Can you work these out from the model? Positions are in its coordinate system, mm. Give positions to 0.01 mm unless a question says otherwise; leave off trailing zeros. Write each loop counter-clockwise with the first axis right and the second up, starting at its lowest first coordinate (ties: lowest second). Pieces come first, ordered by that corner, then holes.
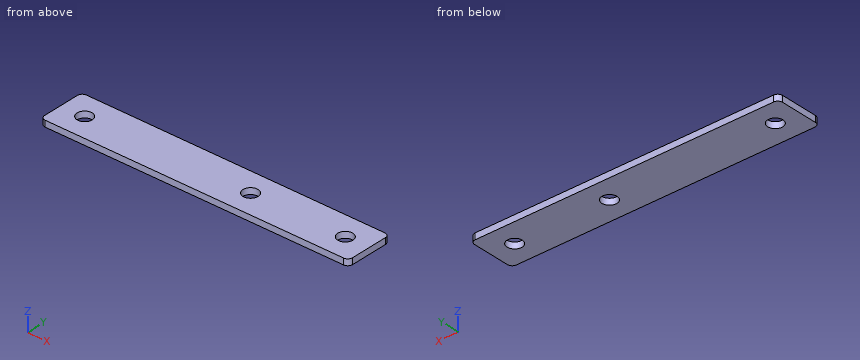
from build123d import *

# Parameters (mm, degrees)
SKETCH_1_W      = 65
SKETCH_1_H      = 10
SKETCH_1_R      = 1.6
EXTRUDE_1_DEPTH = 1.3
FILLET_1_R      = 1


with BuildPart() as part:
    # 草图1 → 凸台-拉伸1 (new body)
    with BuildSketch(Plane.XY):
        with Locations((32.5, 5)):
            Rectangle(SKETCH_1_W, SKETCH_1_H)
        with Locations((60, 5)):
            Circle(SKETCH_1_R, mode=Mode.SUBTRACT)
        with Locations((40, 5)):
            Circle(SKETCH_1_R, mode=Mode.SUBTRACT)
        with Locations((5, 5)):
            Circle(SKETCH_1_R, mode=Mode.SUBTRACT)
    extrude(amount=EXTRUDE_1_DEPTH)

    # 圆角1
    fillet_1_edges = [part.edges().sort_by_distance(p)[0] for p in [
        (0, 10, 0.65),
        (65, 10, 0.65),
        (65, 0, 0.65),
        (0, 0, 0.65),
    ]]
    fillet(fillet_1_edges, radius=FILLET_1_R)


solid = part.part
(1) Imagine slicing it at C-C, the plane z = 0.75. Write out the boundary of the cut face in (x, y).
Returned:
outline: (0, 1) arc R1 ccw to (1, 0) - (64, 0) arc R1 ccw to (65, 1) - (65, 9) arc R1 ccw to (64, 10) - (1, 10) arc R1 ccw to (0, 9) - close; hole circle Ø3.2 at (5, 5); hole circle Ø3.2 at (40, 5); hole circle Ø3.2 at (60, 5)
(2) Imagine slicing it at D-D, the plane x = 60.5. Write out the boundary of the cut face in (y, z).
Returned:
outline: (0, 0) - (3.48, 0) - (3.48, 1.3) - (0, 1.3) - close; (6.52, 0) - (10, 0) - (10, 1.3) - (6.52, 1.3) - close
(3) Imagine slicing it at A-A, the plane x = 5. Write out the boundary of the cut face in (y, z), plus the area to 3 significant figures.
Returned:
outline: (0, 0) - (3.4, 0) - (3.4, 1.3) - (0, 1.3) - close; (6.6, 0) - (10, 0) - (10, 1.3) - (6.6, 1.3) - close
area: 8.84 mm2
(4) If I drill on L1, parallel to Y at x = 5, z = 0.55; L2, parallel to X at y = 0.5, z = 0.7, over which ranges is the centre line in solid material (lowest first)?
Returned:
L1: y = 0 to 3.4, 6.6 to 10
L2: x = 0.13 to 64.87
(5) Imagine slicing it at B-B, the plane y = 5. Write out the boundary of the cut face in (x, z).
Returned:
outline: (0, 0) - (3.4, 0) - (3.4, 1.3) - (0, 1.3) - close; (6.6, 0) - (38.4, 0) - (38.4, 1.3) - (6.6, 1.3) - close; (41.6, 0) - (58.4, 0) - (58.4, 1.3) - (41.6, 1.3) - close; (61.6, 0) - (65, 0) - (65, 1.3) - (61.6, 1.3) - close
